Here's how the part is built. I have some questions about the finished solid (model axes, mm). A direction names the side the tool comes from. Round coordinates to 2 decimals unless told otherwise and drop trailing zeros. Write each loop counter-clockwise with the first axis right and the second up, starting at its lowest first coordinate (ties: lowest second). Pieces come first, ordered by that corner, then holes. Notation, with made-up numbers: (-28, 10.25) -> (-1, 10.25) arc R13 ccw to (-1, 21.25) -> close; hole circle Ø1 at (2.5, 13.25). An arc over 180 degrees is marked (long way). Answer as CSV lines item,"result".
```python
from build123d import *

# Parameters (mm, degrees)
BOSS_EXTRUDE1_DEPTH = 48
FILLET1_R           = 2
SKETCH7_R           = 4.572679887
BOSS_EXTRUDE3_DEPTH = 1
L_EK1_SCALE         = 0.5


with BuildPart() as part:
    # Sketch3 → Boss-Extrude1 (new body)
    with BuildSketch(Plane(origin=(0, 0, 0), x_dir=(1, 0, 0), z_dir=(0, 1, 0))):
        with BuildLine():
            Line((10, 0), (155, 0))
            Line((155, 0), (155, 36))
            Line((155, 36), (10, 36))
            ThreePointArc((10, 36), (2.928932188, 33.071067812), (0, 26))
            Line((0, 26), (0, 10))
            ThreePointArc((0, 10), (2.928932188, 2.928932188), (10, 0))
        make_face()
    extrude(amount=BOSS_EXTRUDE1_DEPTH)

    # Fillet1
    fillet1_edges = [part.edges().sort_by_distance(p)[0] for p in [
        (155, 24, 0),
        (155, 24, -36),
        (2.928932188, 48, -33.071067812),
        (0, 48, -18),
        (2.928932188, 48, -2.928932188),
        (82.5, 48, 0),
        (155, 48, -18),
        (82.5, 0, 0),
        (2.928932188, 0, -2.928932188),
        (0, 0, -18),
        (2.928932188, 0, -33.071067812),
        (82.5, 0, -36),
        (155, 0, -18),
        (82.5, 48, -36),
    ]]
    fillet(fillet1_edges, radius=FILLET1_R)

    # Sketch7 → Boss-Extrude3 (add)
    with BuildSketch(Plane(origin=(0, 48, 0), x_dir=(1, 0, 0), z_dir=(0, 1, 0))):
        with Locations(Location((7.738139678, 28.650889337, 0), (0, 0, 116.659797152))):
            Circle(SKETCH7_R)
        with Locations(Location((7.738139678, 7.349110663, 0), (0, 0, 90))):
            Circle(SKETCH7_R)
    extrude(amount=BOSS_EXTRUDE3_DEPTH)


with BuildPart() as part_1:
    # Ölçek1: scaled about (78.022697694, 24.012137282, -18)
    add(part.part.scale(L_EK1_SCALE).moved(Location((39.011348847, 12.006068641, -9))))


solid = part_1.part
```
1. If I drill on line 1 (Y direction, x = 51, z = -10); line 2 (X direction, y = 29.5, z = -13.5); line 3 (X direction, y = 29.25, z = -23.25), over which ranges is the centre line in solid material (lowest first)?
Numbers:
line 1,"y = 12.01 to 36.01"
line 2,"x = 39.04 to 116.51"
line 3,"x = 39.17 to 116.51"
2. Suppose I cut it at A-A on z = -17.75. Please give me the cut outline in (x, y), and give its area (3 significant figures).
Numbers:
outline,"(39.01, 13.01) arc R1 ccw to (40.01, 12.01) -> (115.51, 12.01) arc R1 ccw to (116.51, 13.01) -> (116.51, 35.01) arc R1 ccw to (115.51, 36.01) -> (40.01, 36.01) arc R1 ccw to (39.01, 35.01) -> close"
area,"1,860 mm^2"
3. Suppose I cut it at B-B on x = 92.5. Please give me the cut outline in (y, z), and give its area (3 significant figures).
Numbers:
outline,"(12.01, -26) arc R1 ccw to (13.01, -27) -> (35.01, -27) arc R1 ccw to (36.01, -26) -> (36.01, -10) arc R1 ccw to (35.01, -9) -> (13.01, -9) arc R1 ccw to (12.01, -10) -> close"
area,"431 mm^2"
4. On a 3-axis mill with a long thin cutter (end or side, diameter ignored), from which of +Z, -Z, +X, -X, +Y, -Y can I reach the whole of each face in a straight line? I mean faces 1 (the face through (43, 36.506, -23)), 2 (the face through (42.194, 36.253, -14.855)). Say none if no direction works.
Numbers:
face 1,"+Z, -Z, +X, -X, +Y"
face 2,"+Y"
5. For pin 1 Ø2 at (x, z) = (64, -20.5) entering from +Y; pin 2 Ø1.5 at (y, z) = (15, -24) entering from -X, each with a flat end and sliding along its axis, tell me the tip position at first contact or that it passes through.
Numbers:
pin 1,"stops at y = 36.01"
pin 2,"stops at x = 39.17"
